```python
from build123d import *

# Parameters (mm, degrees)
SKETCH1_W             = 20
SKETCH1_H             = 20
SKETCH1_R             = 2.25
BOSS_EXTRUDE1_DEPTH   = 8
BOSS_EXTRUDE1_2_DEPTH = 8
BOSS_EXTRUDE2_DEPTH   = 20
FILLET2_R             = 2


with BuildPart() as part:
    # Sketch1 → Boss-Extrude1 (new body)
    with BuildSketch(Plane.XY):
        with Locations((-59.938271605, 0)):
            Rectangle(SKETCH1_W, SKETCH1_H)
        with Locations((-64.938271605, 0)):
            Circle(SKETCH1_R, mode=Mode.SUBTRACT)
    extrude(amount=BOSS_EXTRUDE1_DEPTH)



with BuildPart() as body_2:
    # Sketch1 → Boss-Extrude1 2 (new body)
    with BuildSketch(Plane.XY):
        with Locations((40.061728395, 0)):
            Rectangle(SKETCH1_W, SKETCH1_H)
        with Locations((45.061728395, 0)):
            Circle(SKETCH1_R, mode=Mode.SUBTRACT)
    extrude(amount=BOSS_EXTRUDE1_2_DEPTH)


with BuildPart() as part_1:
    add(part.part)

    add(body_2.part)  # Boss-Extrude2 merges body 2
    # Sketch2 → Boss-Extrude2 (add, through all)
    with BuildSketch(Plane.XZ.offset(10)):
        Polygon((-39.938271605, 25), (20.061728395, 25), (30.061728395, 15), (30.061728395, 8), (38.061728395, 8), (38.061728395, 15), (20.061728395, 33), (-39.938271605, 33), (-57.938271605, 15), (-57.938271605, 8), (-49.938271605, 8), (-49.938271605, 15), align=None)
    extrude(amount=-BOSS_EXTRUDE2_DEPTH)

    # Fillet2
    fillet2_edges = [part_1.edges().sort_by_distance(p)[0] for p in [
        (-69.938271605, 0, 8),
        (-63.938271605, -10, 8),
        (-63.938271605, 10, 8),
        (-44.938271605, 10, 20),
        (-39.938271605, 0, 25),
        (-49.938271605, 0, 15),
        (-57.938271605, 10, 11.5),
        (-57.938271605, 0, 8),
        (-48.938271605, 10, 24),
        (-57.938271605, 0, 15),
        (-9.938271605, 10, 33),
        (-39.938271605, 0, 33),
        (29.061728395, 10, 24),
        (20.061728395, 0, 33),
        (38.061728395, 10, 11.5),
        (38.061728395, 0, 15),
        (38.061728395, 0, 8),
        (30.061728395, 10, 7.5),
        (25.061728395, 10, 20),
        (30.061728395, 0, 15),
        (-9.938271605, 10, 25),
        (20.061728395, 0, 25),
        (-44.938271605, -10, 20),
        (-9.938271605, -10, 25),
        (25.061728395, -10, 20),
        (30.061728395, -10, 7.5),
        (38.061728395, -10, 11.5),
        (29.061728395, -10, 24),
        (-9.938271605, -10, 33),
        (-48.938271605, -10, 24),
        (-57.938271605, -10, 11.5),
        (44.061728395, -10, 8),
        (50.061728395, 0, 8),
        (44.061728395, 10, 8),
        (50.061728395, -10, 4),
        (50.061728395, 10, 4),
        (-49.938271605, -10, 7.5),
        (-69.938271605, -10, 4),
        (-69.938271605, 10, 4),
        (-49.938271605, 10, 7.5),
    ]]
    fillet(fillet2_edges, radius=FILLET2_R)


solid = part_1.part
```
CAD build for the part. Positions are in the model's coordinates, mm. A direction names the side the tool comes from. Coordinates: 2 decimals unless noted, no trailing zeros. Order: outer loops, then holes, each group sorted by start corner. A loop starts at its lowest first (then second) coordinate and runs counter-clockwise, first axis right, second up. Notation, with made-up numbers: M 40,-15.5 L 45,-15.5 A17 ccw 45,17.5 Z; hole C -37.75,23.5 d4. An arc over 180 degrees is marked long. Write each question's results on one line, items separated by ' | '. Start each with the question number.
Q1. Flat gauge pins, fed straight in: P1, Ø8, axis at y = 1.5, z = 11, coming from the +X side; P2, Ø3.5, axis at y = 3.5, z = 13, coming from the +X side; P3, Ø3, axis at x = -47, y = -4.5, coming from the +Z side; P4, Ø10, axis at x = -20, z = 19, coming from the +Y side. Where does each tip first touch, or does it go through?
Q2. Cut at B-B (y = -4.5). List the corners of the cut face in (x, z), then the cut area to 3 significant figures.
Q3. Pull direction X, two halves, no side cores. Call faces 5 (the cylindrical face through (30.663, 9.43, 7.185)), 6 (the cylindrical face through (-69.368, -9.399, 3.042)), 7 (the flat face through (50.062, 0, 3)): +X half, -X half, draft (parallel to the pull), parting line (faces both ways), or undercut.
Q4. Cut at C-C (y = 0). Count the separate pieces of the cut face and the enclosed holes in it, then the cut area to 3 significant figures.
Q5. Drill centre lines: probe 1 along X at (y, z) = (-3.5, 12); probe 2 along X at (y, z) = (-6.5, 3); probe 3 along Y at (x, z) = (21, 26.5). Where is each one in solid material? Low to high. Write a range as from..to.
Q6. Which spindle directions (+Z, -Z, +X, -X, +Y, -Y) get a long thin tool onto all of the face, cutting with end or side? Do faces 1 (the flat face through (42, 0, 8)), 2 (the cylindrical face through (-63.88, -9.4, 7.43)), 3 (the flat face through (-10, 0, 25)), 4 (the cylindrical face through (-63.88, 9.43, 7.4)). Say none if no direction does.
Q7. Cut at A-A (x = -1.5). List the corners of the cut face in (y, z), then the cut area to 3 significant figures.
Found:
1) P1: x = 49.79 | P2: x = 38.06 | P3: z = 27.44 | P4: through
2) outline: M -69.94,0 L -49.94,0 L -49.94,14.17 A2 cw -49.35,15.59 L -40.52,24.41 A2 cw -39.11,25 L 19.23,25 A2 cw 20.65,24.41 L 29.48,15.59 A2 cw 30.06,14.17 L 30.06,0 L 50.06,0 L 50.06,6 A2 ccw 48.06,8 L 40.06,8 A2 cw 38.06,10 L 38.06,14.17 A2 ccw 37.48,15.59 L 20.65,32.41 A2 ccw 19.23,33 L -39.11,33 A2 ccw -40.52,32.41 L -57.35,15.59 A2 ccw -57.94,14.17 L -57.94,10 A2 cw -59.94,8 L -67.94,8 A2 ccw -69.94,6 Z | area: 1,140 mm²
3) face 5: undercut | face 6: -X half | face 7: +X half
4) separate pieces: 3 | enclosed holes: 0 | area: 1,060 mm²
5) probe 1: -57.94..-49.94, 30.06..38.06 | probe 2: -69.94..-49.94, 30.06..50.06 | probe 3: -10..10
6) face 1: +Z, +X, +Y, -Y | face 2: +Z, -X, -Y | face 3: -Z, +Y, -Y | face 4: +Z, -X, +Y
7) outline: M -10,27 A2 ccw -8,25 L 8,25 A2 ccw 10,27 L 10,31 A2 ccw 8,33 L -8,33 A2 ccw -10,31 Z | area: 157 mm²
